Check sheet for the modelled part. Datum: model origin and axes. Units: mm. A direction names the side the tool comes from. Coordinates: 2 decimals unless noted, no trailing zeros. Loops run counter-clockwise (first coordinate to the right, second up) from the corner with the lowest first, then second, coordinate; pieces in that order, holes last. Notation, with made-up numbers: (-16, 21) -> (8, 21) arc R8 cw to (8, 30) -> close; hole circle Ø8 at (-15.5, 25.5). An arc over 180 degrees is marked (long way). Use CSV: the item, a comma, the result in double quotes. Start each with the question number.
1. Thickness scan on L1, parallel to Y at x = 13, z = 7.5; L2, parallel to Z at x = -14, y = 23.5; L3, parallel to X at y = 25, z = 7.5. Record the ranges inside material, lowest first.
2. Set-up check for faces 4 (the face through (10.2, -10.4, 10.7)), 5 (the face through (0, 0, 0)): record each of +Z, -Z, +X, -X, +Y, -Y from which the full face is reachable in a straight line by a thin tool's end or side.
3. Sectioned sample at D-D, the plane x = -14. Record the cut outline in (y, z).
4. Release check for a two-part mould opening along Y. For faces 1 (the face through (-17.996, 27.605, 7.324)), 2 (the face through (-14, 20, 7)), 3 (the face through (10.175, -24.034, 8.021)) record: pulls with the +Y half, pulls with the -Y half, needs draft (parallel to the pull), parting line crosses it, or undercut.
5. Sectioned sample at C-C, the plane z = 7.5. Record the cut outline in (x, y), and give its area (3 significant figures).
6. Sectioned sample at B-B, the plane x = 3.5. Record the cut outline in (y, z), and give its area (3 significant figures).
7. Gauge pin test, flat ends, axial feed: pin 1 (2 mm diameter, centred on x = -15, z = 2.5, fed in from -Y); pin 2 (2.5 mm diameter, centred on x = -13, z = 7, fed in from +Y); pin 3 (4 mm diameter, centred on y = -29, z = 9, fed in from +X); pin 4 (1.5 mm diameter, centred on x = -2.5, y = 17, fed in from -Z). Record the tip position at first contact, or that the pin passes through.
8. Sectioned sample at A-A, the plane y = -28. Record the cut outline in (x, z).
```python
from build123d import *

# Parameters (mm, degrees)
SZKIC1_W                    = 45
SZKIC1_H                    = 70
DODANIE_WYCI_GNI_CIE1_DEPTH = 15
SZKIC3_R                    = 4
WYTNIJ_WYCI_GNI_CIE1_DEPTH  = 15
SFAZOWANIE1_SIZE            = 12
SZKIC4_R                    = 4
WYTNIJ_WYCI_GNI_CIE2_DEPTH  = 25


with BuildPart() as part:
    # Szkic1 → Dodanie-wyciągnięcie1 (new body)
    with BuildSketch(Plane.XY):
        Rectangle(SZKIC1_W, SZKIC1_H)
    extrude(amount=DODANIE_WYCI_GNI_CIE1_DEPTH)

    # Szkic3 → Wytnij-wyciągnięcie1 (cut)
    with BuildSketch(Plane(origin=(0, 35, 0), x_dir=(1, 0, 0), z_dir=(0, 1, 0))):
        with Locations((-14, -7.5)):
            Circle(SZKIC3_R)
    extrude(amount=-WYTNIJ_WYCI_GNI_CIE1_DEPTH, mode=Mode.SUBTRACT)

    # Sfazowanie1
    sfazowanie1_edges = [part.edges().sort_by_distance(p)[0] for p in [
        (-22.5, -35, 7.5),
    ]]
    chamfer(sfazowanie1_edges, length=SFAZOWANIE1_SIZE)

    # Szkic4 → Wytnij-wyciągnięcie2 (cut)
    with BuildSketch(Plane(origin=(22.5, 0, 0), x_dir=(0, 0, -1), z_dir=(1, 0, 0))):
        with Locations((-7.5, -28)):
            Circle(SZKIC4_R)
        with Locations((-7.5, -8)):
            Circle(SZKIC4_R)
    extrude(amount=-WYTNIJ_WYCI_GNI_CIE2_DEPTH, mode=Mode.SUBTRACT)


solid = part.part
```
Completed:
1,L1,"-35 to -32, -24 to -12, -4 to 35"
1,L2,"0 to 3.5, 11.5 to 15"
1,L3,"-22.5 to -18, -10 to 22.5"
2,face 4,"+X"
2,face 5,"-Z, +X, -X, +Y, -Y"
3,outline,"(-31.5, 0) -> (35, 0) -> (35, 3.5) -> (20, 3.5) -> (20, 11.5) -> (35, 11.5) -> (35, 15) -> (-31.5, 15) -> close"
4,face 1,"needs draft"
4,face 2,"pulls with the +Y half"
4,face 3,"undercut"
5,outline,"(-22.5, -23) -> (-10.5, -35) -> (22.5, -35) -> (22.5, -32) -> (-2.5, -32) -> (-2.5, -24) -> (22.5, -24) -> (22.5, -12) -> (-2.5, -12) -> (-2.5, -4) -> (22.5, -4) -> (22.5, 35) -> (-10, 35) -> (-10, 20) -> (-18, 20) -> (-18, 35) -> (-22.5, 35) -> close"
5,area,"2,560 mm²"
6,outline,"(-35, 0) -> (35, 0) -> (35, 15) -> (-35, 15) -> close; hole circle Ø8 at (-28, 7.5); hole circle Ø8 at (-8, 7.5)"
6,area,"949 mm²"
7,pin 1,"y = -31.5"
7,pin 2,"y = 20"
7,pin 3,"x = -2.5"
7,pin 4,"z = 0"
8,outline,"(-17.5, 0) -> (22.5, 0) -> (22.5, 3.5) -> (-2.5, 3.5) -> (-2.5, 11.5) -> (22.5, 11.5) -> (22.5, 15) -> (-17.5, 15) -> close"
